Model file for the job. Use its own axes, mm. Face numbers are marked on the shaded views. A direction names the side the tool comes from. Round coordinates to 2 decimals unless told otherwise and drop trailing zeros. Order: outer loops, then holes, each group sorted by start corner. A loop starts at its lowest first (then second) coordinate and runs counter-clockwise, first axis right, second up. Notation, with made-up numbers: (79, 17.25) - (110, 17.25) arc R18 ccw to (110, 31.25) - close; hole circle Ø10 at (60, 16.25). An arc over 180 degrees is marked (long way). Write item = value, one per line. Start each with the question number.
from build123d import *

# Parameters (mm, degrees)
BOSS_EXTRUDE2_DEPTH      = 10
CUT_EXTRUDE2_DEPTH       = 90.877694674
CUT_EXTRUDE2_DEPTH_BACK  = 90.877694674
SKETCH5_W                = 11
SKETCH5_H                = 67.407766248
CUT_EXTRUDE3_DEPTH       = 87.446515257
CUT_EXTRUDE3_DEPTH_BACK  = 87.446515257
SKETCH16_R               = 1.85
FILLET16_R               = 15
CUT_EXTRUDE20_DEPTH      = 92.021975369
CUT_EXTRUDE20_DEPTH_BACK = 92.021975369
SKETCH45_R               = 1.85
SKETCH52_W               = 15
SKETCH52_H               = 10
BOSS_EXTRUDE25_DEPTH     = 4
FILLET17_R               = 10
FILLET18_R               = 2
SKETCH53_R               = 1.9
CUT_EXTRUDE25_DEPTH      = 10
SKETCH55_W               = 0.5
SKETCH55_H               = 4
CUT_EXTRUDE28_DEPTH      = 10
SKETCH56_W               = 10
SKETCH56_H               = 4
BOSS_EXTRUDE26_DEPTH     = 36
SKETCH57_R               = 1.9
CUT_EXTRUDE29_DEPTH      = 36
SKETCH59_W               = 5
SKETCH59_H               = 10
CUT_EXTRUDE31_DEPTH      = 4
CUT_EXTRUDE32_DEPTH      = 91.05553843
CUT_EXTRUDE32_DEPTH_BACK = 91.05553843
SKETCH60_R               = 2


with BuildPart() as part:
    # Sketch2 → Boss-Extrude2 (new body)
    with BuildSketch(Plane.XY):
        Polygon((18, -3), (33, -3), (33, 43), (-3, 43), (-3, -3), (11, -3), (11, -83), (18, -83), align=None)
        Polygon((15, 0), (30, 0), (30, 40), (0, 40), (0, 0), (14, 0), (14, -80), (15, -80), align=None, mode=Mode.SUBTRACT)
    extrude(amount=BOSS_EXTRUDE2_DEPTH)

    # Sketch5 → Cut-Extrude2 (cut, two sides: drawn at the far end of the back side and taken through both)
    with BuildSketch(Plane.XY.offset(10).offset(-CUT_EXTRUDE2_DEPTH_BACK)):
        with Locations((9.5, -51.703883124)):
            Rectangle(SKETCH5_W, SKETCH5_H)
    extrude(amount=CUT_EXTRUDE2_DEPTH + CUT_EXTRUDE2_DEPTH_BACK, mode=Mode.SUBTRACT)

    # Sketch16 → Cut-Extrude3 (cut, two sides: drawn at the far end of the back side and taken through both)
    with BuildSketch(Plane.ZY.offset(-11).offset(-CUT_EXTRUDE3_DEPTH_BACK)):
        with Locations((5, -10.5)):
            Circle(SKETCH16_R)
    extrude(amount=CUT_EXTRUDE3_DEPTH + CUT_EXTRUDE3_DEPTH_BACK, mode=Mode.SUBTRACT)

    # Fillet16
    # the kernel refuses this fillet: 15 mm, written as the material it adds along each edge
    with BuildSketch(Plane(origin=(0, 40, 0), x_dir=(0, -1, 0), z_dir=(0, 0, 1)), Plane(origin=(30, 40, 0), x_dir=(-1, 0, 0), z_dir=(0, 0, 1)), Plane(origin=(30, 0, 0), x_dir=(0, 1, 0), z_dir=(0, 0, 1))) as fillet16_piece_1:
        with BuildLine():
            CenterArc((FILLET16_R, FILLET16_R), FILLET16_R, 180, 90)
            Line((0, FILLET16_R), (-FILLET16_R * 0.02, FILLET16_R))
            Line((-FILLET16_R * 0.02, FILLET16_R), (-FILLET16_R * 0.02, -FILLET16_R * 0.02))
            Line((-FILLET16_R * 0.02, -FILLET16_R * 0.02), (FILLET16_R, -FILLET16_R * 0.02))
            Line((FILLET16_R, -FILLET16_R * 0.02), (FILLET16_R, 0))
        make_face()
    extrude(amount=10)
    with BuildSketch(Plane(origin=(0, 0, 0), x_dir=(1, 0, 0), z_dir=(0, 0, 1))) as fillet16_piece_2:
        with BuildLine():
            CenterArc((15, 14.966629547), FILLET16_R, 180, 86.177446271)
            Line((0, 14.966629547), (-0.3, 14.966629547))
            Line((-0.3, 14.966629547), (-0.3, 0))
            Line((-0.3, 0), (0, -0.3))
            ThreePointArc((0, -0.3), (7, -0.3), (13.98, -0.299332591))
            Line((13.98, -0.299332591), (14, 0))
        make_face()
    extrude(amount=10)

    # Sketch45 → Cut-Extrude20 (cut, two sides: drawn at the far end of the back side and taken through both)
    with BuildSketch(Plane.ZY.offset(3).offset(-CUT_EXTRUDE20_DEPTH_BACK)):
        with Locations((5, 20)):
            Circle(SKETCH45_R)
    extrude(amount=CUT_EXTRUDE20_DEPTH + CUT_EXTRUDE20_DEPTH_BACK, mode=Mode.SUBTRACT)

    # Sketch52 → Boss-Extrude25 (add)
    with BuildSketch(Plane.XZ.offset(83)):
        with Locations((10.5, 5)):
            Rectangle(SKETCH52_W, SKETCH52_H)
    extrude(amount=BOSS_EXTRUDE25_DEPTH)

    # Fillet17
    fillet17_edges = [part.edges().sort_by_distance(p)[0] for p in [
        (-3, -3, 5),
        (33, -3, 5),
    ]]
    fillet(fillet17_edges, radius=FILLET17_R)

    # Fillet18
    fillet18_edges = [part.edges().sort_by_distance(p)[0] for p in [
        (18, -87, 5),
    ]]
    fillet(fillet18_edges, radius=FILLET18_R)

    # Sketch53 → Cut-Extrude25 (cut)
    with BuildSketch(Plane.XZ.offset(87)):
        with Locations(Location((8, 5, 0), (0, 0, 270))):
            Circle(SKETCH53_R)
    extrude(amount=-CUT_EXTRUDE25_DEPTH, mode=Mode.SUBTRACT)

    # Sketch55 → Cut-Extrude28 (cut)
    with BuildSketch(Plane.ZY.offset(-3)):
        with Locations((0.25, -85)):
            Rectangle(SKETCH55_W, SKETCH55_H)
    extrude(amount=-CUT_EXTRUDE28_DEPTH, mode=Mode.SUBTRACT)

    # Sketch56 → Boss-Extrude26 (add)
    with BuildSketch(Plane.ZY.offset(3)):
        with Locations((5, 45)):
            Rectangle(SKETCH56_W, SKETCH56_H)
    extrude(amount=-BOSS_EXTRUDE26_DEPTH)

    # Sketch57 → Cut-Extrude29 (cut)
    with BuildSketch(Plane(origin=(0, 47, 0), x_dir=(1, 0, 0), z_dir=(0, 1, 0))):
        with Locations(Location((15, -5, 0), (0, 0, 270))):
            Circle(SKETCH57_R)
    extrude(amount=-CUT_EXTRUDE29_DEPTH, mode=Mode.SUBTRACT)

    # Sketch59 → Cut-Extrude31 (cut)
    with BuildSketch(Plane(origin=(0, 47, 0), x_dir=(1, 0, 0), z_dir=(0, 1, 0))):
        with Locations((15, -5)):
            Rectangle(SKETCH59_W, SKETCH59_H)
    extrude(amount=-CUT_EXTRUDE31_DEPTH, mode=Mode.SUBTRACT)

    # Sketch60 → Cut-Extrude32 (cut, two sides: drawn at the far end of the back side and taken through both)
    with BuildSketch(Plane(origin=(18, 0, 0), x_dir=(0, 0, -1), z_dir=(1, 0, 0)).offset(-CUT_EXTRUDE32_DEPTH_BACK)):
        with Locations((-5, -10.5)):
            Circle(SKETCH60_R)
    extrude(amount=CUT_EXTRUDE32_DEPTH + CUT_EXTRUDE32_DEPTH_BACK, mode=Mode.SUBTRACT)


solid = part.part
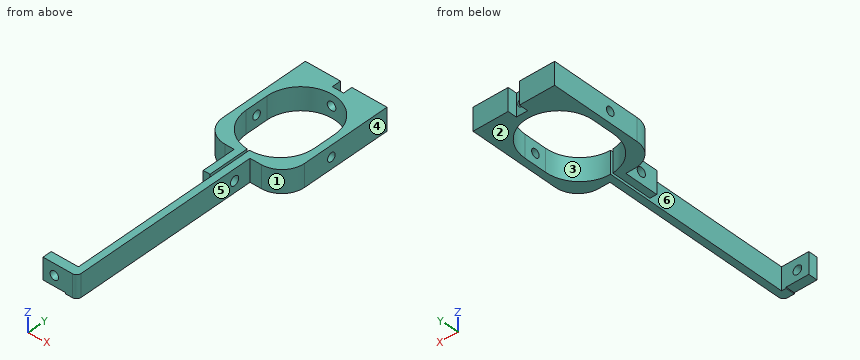
Item 1: Saw through at B-B, the plane y = 5.5. Give the cut face in (x, z), then the cut area to 3 significant figures.
Item 2: Saw through at A-A, the plane y = 20. Give the cut face in (x, z), then the cut area to 3 significant figures.
Item 3: Probe L1, parallel to Z at x = -1, y = 20; L2, parallel to Y at x = 6, z = 2.5; L3, parallel to X at y = 22, z = 6. List the from-to ranges inside material, lowest first.
Item 4: Drop flat-ended pins along their axis: pin 1 (6 mm diameter, centred on y = 20, z = 5, fed in from +X); pin 2 (1 mm diameter, centred on y = -65, z = 8.5, fed in from -X); pin 3 (1.2 mm diameter, centred on y = -85, z = 6.5, fed in from -X); pin 4 (5 mm diameter, centred on y = -35.5, z = 7, fed in from +X). Give the stop position or say it passes through.
Item 5: Mould opens along X. For the marked faces 1, 2 and 3 say: +X half, -X half, draft (parallel to the pull), parting line (faces both ways), or undercut.
Item 6: Saw through at C-C, the plane z = 5. Give the number of separate pieces and of enclosed holes in the cut face, then the cut area to 3 significant figures.
Item 7: Which spindle directions (+Z, -Z, +X, -X, +Y, -Y) get a long thin tool onto all of the face, cutting with end or side? Do the marked faces 4, 5 and 6. Say none if no direction does.
Item 8: Saw through at D-D, the plane y = -10.5. Give the cut face in (x, z), then the cut area to 3 significant figures.
Check sheet entries:
q1.outline = (-2.89, 0) - (3.36, 0) - (3.36, 10) - (-2.89, 10) - close; (26.61, 0) - (32.89, 0) - (32.89, 10) - (26.61, 10) - close
q1.area = 125 mm2
q2.outline = (-3, 0) - (0, 0) - (0, 3.15) - (-3, 3.15) - close; (-3, 6.85) - (0, 6.85) - (0, 10) - (-3, 10) - close; (30, 0) - (33, 0) - (33, 3.15) - (30, 3.15) - close; (30, 6.85) - (33, 6.85) - (33, 10) - (30, 10) - close
q2.area = 37.8 mm2
q3.L1 = 0 to 3.15, 6.85 to 10
q3.L2 = -87 to -83, -2.95 to 2.97, 37 to 47
q3.L3 = -3 to 0, 30 to 33
q4.pin_1 = 33
q4.pin_2 = 15
q4.pin_3 = 3
q4.pin_4 = 18
q5.face_1 = +X half
q5.face_2 = draft
q5.face_3 = undercut
q6.separate_pieces = 7
q6.enclosed_holes = 0
q6.area = 998 mm2
q7.face_4 = +Z, -Z, +X, +Y, -Y
q7.face_5 = +Z, -Z, +X, -Y
q7.face_6 = +Z, -Z
q8.outline = (11, 0) - (14, 0) - (14, 3) - (11, 3) - close; (11, 7) - (14, 7) - (14, 10) - (11, 10) - close; (15, 0) - (18, 0) - (18, 3) - (15, 3) - close; (15, 7) - (18, 7) - (18, 10) - (15, 10) - close
q8.area = 36.0 mm2
